Build history of the part. All positions in model axes, mm. A direction names the side the tool comes from. Give positions to 0.01 mm unless a question says otherwise; leave off trailing zeros. Order: outer loops, then holes, each group sorted by start corner. A loop starts at its lowest first (then second) coordinate and runs counter-clockwise, first axis right, second up. Notation, with made-up numbers: (-26, -15.75) - (8, -15.75) arc R19 cw to (8, -7.75) - close; hole circle Ø11 at (25, 12.25). An arc over 180 degrees is marked (long way). Use a Markdown table: item, result. Add a question column.
(1) Wall check: line 1 (Z direction, x = 0, y = 3.8); line 2 (Z direction, x = 72, y = 4.8). Give the ranges that are in metal, low to high.
(2) Which spindle directions (+Z, -Z, +X, -X, +Y, -Y) get a long thin tool onto all of the face, cutting with end or side? Do faces 1 (the face through (52, 3, -69)), 2 (the face through (-52, 3, 69)), 3 (the face through (-69, 3, -52)), 4 (the face through (35, 3, 72)). Say none if no direction does.
(3) Slice it at A-A (y = 3.2). Write the cut outline in (x, z).
(4) Slice it at B-B (x = 58). Write the cut outline in (y, z).
(5) Flat gauge pins, fed straight in: pin 1 (1.8 mm diameter, centred on x = -54, y = 3.5, fed in from +Z); pin 2 (2 mm diameter, centred on y = 1, z = -39, fed in from +X); pin 3 (1.8 mm diameter, centred on x = -71, y = 3.5, fed in from -Z). Where does each tip first touch, or does it go through?
(6) Slice it at C-C (z = 53). Write the cut outline in (x, y), then the cut area to 3 significant figures.
from build123d import *

# Parameters (mm, degrees)
SKETCH1_R           = 1.5
BOSS_EXTRUDE1_DEPTH = 6


with BuildPart() as part:
    # Sketch1 → Boss-Extrude1 (new body)
    with BuildSketch(Plane(origin=(0, 0, 0), x_dir=(1, 0, 0), z_dir=(0, 1, 0))):
        Polygon((69, 69), (35, 69), (35, 75), (-35, 75), (-35, 69), (-69, 69), (-69, 35), (-75, 35), (-75, -35), (-69, -35), (-69, -69), (-35, -69), (-35, -75), (35, -75), (35, -69), (69, -69), (69, -35), (75, -35), (75, 35), (69, 35), align=None)
        with Locations((0, 72)):
            Circle(SKETCH1_R, mode=Mode.SUBTRACT)
        with Locations((-72, 0)):
            Circle(SKETCH1_R, mode=Mode.SUBTRACT)
        with Locations((72, 0)):
            Circle(SKETCH1_R, mode=Mode.SUBTRACT)
        with Locations((0, -72)):
            Circle(SKETCH1_R, mode=Mode.SUBTRACT)
    extrude(amount=BOSS_EXTRUDE1_DEPTH)


solid = part.part
Solution:
| question | item | result |
|---|---|---|
| 1 | line 1 | -75 to -73.5, -70.5 to 70.5, 73.5 to 75 |
| 1 | line 2 | -35 to -1.5, 1.5 to 35 |
| 2 | face 1 | -Z, +X, +Y, -Y |
| 2 | face 2 | +Z, -X, +Y, -Y |
| 2 | face 3 | -Z, -X, +Y, -Y |
| 2 | face 4 | +Z, +X, +Y, -Y |
| 3 | outline | (-75, -35) - (-69, -35) - (-69, -69) - (-35, -69) - (-35, -75) - (35, -75) - (35, -69) - (69, -69) - (69, -35) - (75, -35) - (75, 35) - (69, 35) - (69, 69) - (35, 69) - (35, 75) - (-35, 75) - (-35, 69) - (-69, 69) - (-69, 35) - (-75, 35) - close; hole circle Ø3 at (-72, 0); hole circle Ø3 at (0, -72); hole circle Ø3 at (0, 72); hole circle Ø3 at (72, 0) |
| 4 | outline | (0, -69) - (6, -69) - (6, 69) - (0, 69) - close |
| 5 | pin 1 | z = 69 |
| 5 | pin 2 | x = 69 |
| 5 | pin 3 | z = -35 |
| 6 | outline | (-69, 0) - (69, 0) - (69, 6) - (-69, 6) - close |
| 6 | area | 828 mm2 |
